Geometry check sheet. Reference: the model listing, model coordinates, mm. Coordinates: 2 decimals unless noted, no trailing zeros. Write each loop counter-clockwise with the first axis right and the second up, starting at its lowest first coordinate (ties: lowest second). Pieces come first, ordered by that corner, then holes. Notation, with made-up numbers: (-39, -40) -> (20, -40) arc R28 ccw to (20, -4) -> close; hole circle Ø4 at (73.25, -4.75). An arc over 180 degrees is marked (long way). One line per question, with ' | ' between items.
```python
from build123d import *

# Parameters (mm, degrees)
SKETCH2_R             = 9.144
THICKER_SECTION_DEPTH = 38.1
SKETCH3_R             = 8.128
SMALLER_SECTION_DEPTH = 124.46
SKETCH4_R             = 2
CUT_EXTRUDE1_DEPTH    = 19.05


with BuildPart() as part:
    # Sketch2 → Thicker Section (new body)
    with BuildSketch(Plane.XY):
        with Locations(Location((0, 0, 0), (0, 0, 180))):
            Circle(SKETCH2_R)
    extrude(amount=THICKER_SECTION_DEPTH)

    # Sketch3 → Smaller  Section (add)
    with BuildSketch(Plane.XY.offset(38.1)):
        with Locations(Location((0, 0, 0), (0, 0, 180))):
            Circle(SKETCH3_R)
    extrude(amount=SMALLER_SECTION_DEPTH)

    # Sketch4 → Cut-Extrude1 (cut)
    with BuildSketch(Plane.XY.offset(162.56)):
        Circle(SKETCH4_R)
    extrude(amount=-CUT_EXTRUDE1_DEPTH, mode=Mode.SUBTRACT)


solid = part.part
```
(1) Cross-section at A-A (x = 0). Record the cut outline in (y, z), plus the area to 3 significant figures.
Answers below:
outline: (-9.14, 0) -> (9.14, 0) -> (9.14, 38.1) -> (8.13, 38.1) -> (8.13, 162.56) -> (2, 162.56) -> (2, 143.51) -> (-2, 143.51) -> (-2, 162.56) -> (-8.13, 162.56) -> (-8.13, 38.1) -> (-9.14, 38.1) -> close | area: 2,640 mm²
(2) Material ranges on line 1 (Y direction, x = 0, z = 149.5); line 2 (X direction, y = -0.25, z = 135.5); line 3 (Z direction, x = -7.25, y = -3.75), recorded low to high.
Answers below:
line 1: y = -8.13 to -2, 2 to 8.13 | line 2: x = -8.12 to 8.12 | line 3: z = 0 to 38.1
(3) Depth check by flat-ended pin: P1, Ø2, axis at x = 0.5, y = 0.5, coming from the +Z side; P2, Ø6, axis at y = -2, z = 127.5, coming from the -X side; P3, Ø8, axis at x = 6.5, z = 95.5, coming from the -Y side. Enter the tip coordinate at first touch or a pass-through.
Answers below:
P1: stops at z = 143.51 | P2: stops at x = -8.13 | P3: stops at y = -7.73
(4) Draft check along Y on faces 1 (the face through (8.2, 1.3, 38.1)), 2 (the face through (0, -2, 153)), 3 (the face through (0, 0, 143.51)), 4 (the face through (1.762, 7.935, 99.459)). Enter one of: pulls with the +Y half, pulls with the -Y half, needs draft (parallel to the pull), parting line crosses it, or undercut.
Answers below:
face 1: needs draft | face 2: undercut | face 3: undercut | face 4: parting line crosses it
(5) Cross-section at C-C (z = 27). Record the cut outline in (x, y), plus the area to 3 significant figures.
Answers below:
outline: circle Ø18.29 at (0, 0) | area: 263 mm²
(6) Cross-section at D-D (y = -6.75). Record the cut outline in (x, z).
Answers below:
outline: (-6.17, 0) -> (6.17, 0) -> (6.17, 38.1) -> (4.53, 38.1) -> (4.53, 162.56) -> (-4.53, 162.56) -> (-4.53, 38.1) -> (-6.17, 38.1) -> close
